Autodesk Inventor part; units mm, degrees
ref_plane "YZ Plane" through (0, 0, 0) normal (1, 0, 0) x (0, 1, 0)
ref_plane "XZ Plane" through (0, 0, 0) normal (0, 1, 0) x (-1, 0, 0)
ref_plane "XY Plane" through (0, 0, 0) normal (0, 0, 1) x (1, 0, 0)
sketch "Boceto1" plane through (0, 0, 0) normal (0, 1, 0) x (-1, 0, 0)
  line L0 (-15, -50) -> (15, -50)
  line L1 (20, -45) -> (20, 45)
  line L2 (15, 50) -> (-15, 50)
  line L3 (-20, 45) -> (-20, -45)
  arc A0 (-15, 50) -> (-20, 45) centre (-15, 45) ccw
  arc A1 (-20, -45) -> (-15, -50) centre (-15, -45) ccw
  arc A2 (15, -50) -> (20, -45) centre (15, -45) ccw
  arc A3 (20, 45) -> (15, 50) centre (15, 45) ccw
  circle A4 centre (0, 28.75) radius 10
  circle A5 centre (0.1077, -28.75) radius 10
  point P0 (0, 0)
  dimension "d3" = 5
  dimension "d4" = 5
  dimension "d5" = 5
  dimension "d6" = 5
  dimension "d7" = 20
  dimension "d8" = 20
  dimension "d10" = 28.75
  dimension "d11" = 28.75
extrude "Extrusión1" add sketch "Boceto1" along normal blind 10
extrude "Extrusión2" add sketch "Boceto1" along normal blind 12 contours A4 | A5
sketch "Boceto2" plane through (0, 12, 28.75) normal (0, 1, 0) x (1, 0, 0)
  circle A0 centre (0, 0) radius 7.5
  circle A1 centre (-0.1077, 57.5) radius 7.5
  circle A2 centre (-0.1077, 57.5) radius 10
  circle A3 centre (0, 0) radius 10
  point P0 (0, 28.75)
  dimension "d16" = 15
  dimension "d17" = 15
  dimension "d26" = 2.5
extrude "Extrusión3" add sketch "Boceto2" along normal blind 15 contours A0 | A1
sketch "Boceto3" plane through (0, 27, 28.75) normal (0, 1, 0) x (1, 0, 0)
  circle A0 centre (0, 0) radius 7.5
  circle A1 centre (0, 0) radius 10
  circle A2 centre (-0.1077, 57.5) radius 10
  circle A3 centre (-0.1077, 57.5) radius 10
  point P0 (0, 28.75)
  dimension "d20" = 20
  dimension "d21" = 20
extrude "Extrusión4" add sketch "Boceto3" along normal blind 2 contours A0 | A1 | A2
fillet "Empalme1" radius 1.5 4 edges at (10, 12, 28.75) (-10, 27, 28.75) (9.8923, 12, -28.75) (-10.1077, 27, -28.75)
properties part number "Soporte Engrane"
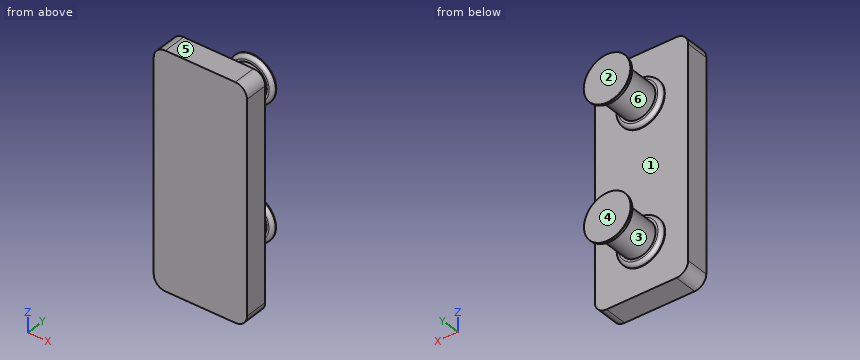
Model file for the job. Use its own axes, mm. Face numbers are marked on the shaded views. A direction names the side the tool comes from. Give positions to 0.01 mm unless a question says otherwise; leave off trailing zeros. Write each loop counter-clockwise with the first axis right and the second up, starting at its lowest first coordinate (ties: lowest second). Pieces come first, ordered by that corner, then holes. Notation, with made-up numbers: (-40, 5) - (-28, 5) arc R14 ccw to (-28, 26) - close; hole circle Ø9 at (-30, -9.5). An arc over 180 degrees is marked (long way). One line per question, with ' | ' between items. Start each with the question number.
(1) Slice it at D-D on z = 1. Write the cut outline in (x, y), plus the area to 3 significant figures.
(2) Slice it at C-C on x = 12. Write the cut outline in (y, z), plus the area to 3 significant figures.
(3) Wall check: line 1 along Y through (x, z) = (-4, -14); line 2 along Z through (x, y) = (-6.5, 14.25); line 3 along Z through (x, y) = (-5, 24.5). Give the ranges that are in metal, low to high. Write a range as from..to.
(4) Pin check, flat tips, straight feed: P1, Ø4, axis at x = -6.5, z = -2.5, coming from the +Y side; P2, Ø4, axis at y = 21.5, z = -39.5, coming from the -X side. Stop position of each tip, or through.
(5) Slice it at A-A on z = 28.75. Write the cut outline in (x, y), plus the area to 3 significant figures.
(6) Two-plate mould, pull along Z, no slides. Class the marked faces 4, 5 and 6: +Z half, -Z half, draft (parallel to the pull), parting line (faces both ways), or undercut.
(7) 3-axis set-ups, long thin cutter, end or side, ignore diameter. For the marked faces 1, 2 and 3: which of +Z, -Z, +X, -X, +Y, -Y reach the whole face in a straight line?
(8) Slice it at B-B on y = 15. Write the cut outline in (x, z).
Results below:
1) outline: (-20, 0) - (20, 0) - (20, 10) - (-20, 10) - close | area: 400 mm^2
2) outline: (0, -50) - (10, -50) - (10, 50) - (0, 50) - close | area: 1,000 mm^2
3) line 1: 0..10 | line 2: -32.67..-24.83, 25.01..32.49 | line 3: -34.43..-23.07, 23.16..34.34
4) P1: y = 10 | P2: through
5) outline: (-20, 0) - (20, 0) - (20, 10) - (10, 10) - (10, 10.5) arc R1.5 ccw to (8.5, 12) - (7.5, 12) - (7.5, 27) - (8.5, 27) arc R1.5 ccw to (10, 28.5) - (10, 29) - (-10, 29) - (-10, 28.5) arc R1.5 ccw to (-8.5, 27) - (-7.5, 27) - (-7.5, 12) - (-8.5, 12) arc R1.5 ccw to (-10, 10.5) - (-10, 10) - (-20, 10) - close | area: 703 mm^2
6) face 4: draft | face 5: +Z half | face 6: undercut
7) face 1: +Y | face 2: +Z, -Z, +X, -X, +Y | face 3: none
8) outline: circle Ø15 at (-0.11, -28.75); circle Ø15 at (0, 28.75)
